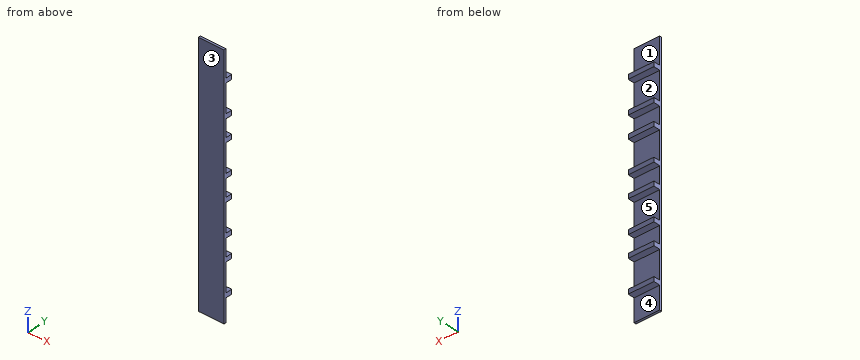
```python
from build123d import *

# Parameters (mm, degrees)
SKETCH2_W           = 5.7
SKETCH2_H           = 0.5
BOSS_EXTRUDE1_DEPTH = 55.1
SKETCH3_W           = 5.7
SKETCH3_H           = 1
BOSS_EXTRUDE2_DEPTH = 1.45
LPATTERN1_COUNT     = 4
LPATTERN1_PITCH     = 12


with BuildPart() as part:
    # Sketch2 → Boss-Extrude1 (new body)
    with BuildSketch(Plane.XY):
        with Locations((2.85, 0.25)):
            Rectangle(SKETCH2_W, SKETCH2_H)
    extrude(amount=BOSS_EXTRUDE1_DEPTH)

    # Sketch3 → Boss-Extrude2 (add)
    with BuildSketch(Plane(origin=(0, 0.5, 0), x_dir=(1, 0, 0), z_dir=(0, 1, 0))):
        with Locations((2.85, -5.5)):
            Rectangle(SKETCH3_W, SKETCH3_H)
        with Locations((2.85, -12.7)):
            Rectangle(SKETCH3_W, SKETCH3_H)
    boss_extrude2 = extrude(amount=BOSS_EXTRUDE2_DEPTH)

    # LPattern1: Boss-Extrude2 ×4
    with Locations(*[(0, 0, i * LPATTERN1_PITCH) for i in range(1, LPATTERN1_COUNT)]):
        add(boss_extrude2)


solid = part.part
```
Build history of the part. All positions in model axes, mm. Face numbers are marked on the shaded views. A direction names the side the tool comes from. Round coordinates to 2 decimals unless told otherwise and drop trailing zeros. Loops run counter-clockwise (first coordinate to the right, second up) from the corner with the lowest first, then second, coordinate; pieces in that order, holes last.
Item 1: Saw through at A-A (y = 1.55). State how many separate pieces and enclosed holes the cut face has, then the cut area to 3 significant figures.
Item 2: Which spindle directions (+Z, -Z, +X, -X, +Y, -Y) get a long thin tool onto all of the face, cutting with end or side? Do the marked faces 3, 4 and 5. Say none if no direction does.
Item 3: Drill centre line: line 1 along Y through (x, z) = (4.05, 24). Where is it in solid material? Low to high.
Item 4: Two-plate mould, pull along Z, no slides. Class the marked faces 1 and 2: released by +Z, released by -Z, zero draft, split by the parting line, or undercut.
Item 5: Saw through at B-B (z = 34.5). List the corners of the cut face in (x, y), then the cut area to 3 significant figures.
Item 6: Pin check, flat tips, straight feed: P1, Ø1.7, axis at x = 4, z = 46, coming from the +Y side; P2, Ø0.7, axis at x = 2.5, y = 1.5, coming from the +Z side. Stop position of each tip, or through.
Worked answers:
1. separate pieces: 8
1. enclosed holes: 0
1. area: 45.6 mm2
2. face 3: +Z, -Z, +X, -X, -Y
2. face 4: -Z, +X, -X, +Y
2. face 5: +X, -X, +Y
3. line 1: y = 0 to 0.5
4. face 1: zero draft
4. face 2: undercut
5. outline: (0, 0) - (5.7, 0) - (5.7, 0.5) - (0, 0.5) - close
5. area: 2.85 mm2
6. P1: stops at y = 0.5
6. P2: stops at z = 49.2
